Input: dimensioned drawing with shaded views. Units: mm. Origin: part minimum x, y, z. Give positions to 0.01 mm unless a question says otherwise; leave off trailing zeros. Write each loop counter-clockwise with the first axis right and the second up, starting at its lowest first coordinate (ties: lowest second). Pieces come first, ordered by that corner, then holes.
Q1. Section A-A (y = 19). Return the cut outline in (x, z).
Q2. Pin query (flat end, axial travel): pin 1 Ø4 at (y, z) = (28.5, 11.5) entering from -X; pin 2 Ø5 at (y, z) = (26.5, 7.5) entering from -X; pin 3 Ø5 at (x, z) = (24.5, 17) entering from -Y. Return the tip coordinate at first contact, or that it passes through.
Q3. Mould query, pull axis Y, two halves, no side actions, for the marked faces 1, 2 and 3. Classes: +Y half, -Y half, draft (parallel to the pull), parting line (faces both ways), or undercut.
Q4. Line query: line 1 (Y direction, x = 19, z = 6.75); line 2 (Y direction, x = 14.5, z = 9.25); line 3 (X direction, y = 23, z = 12.5). Output: solid intervals per line, ascending.
Q5. Section C-C (z = 11.5). Return the cut outline in (x, y), plus the area to 3 significant figures.
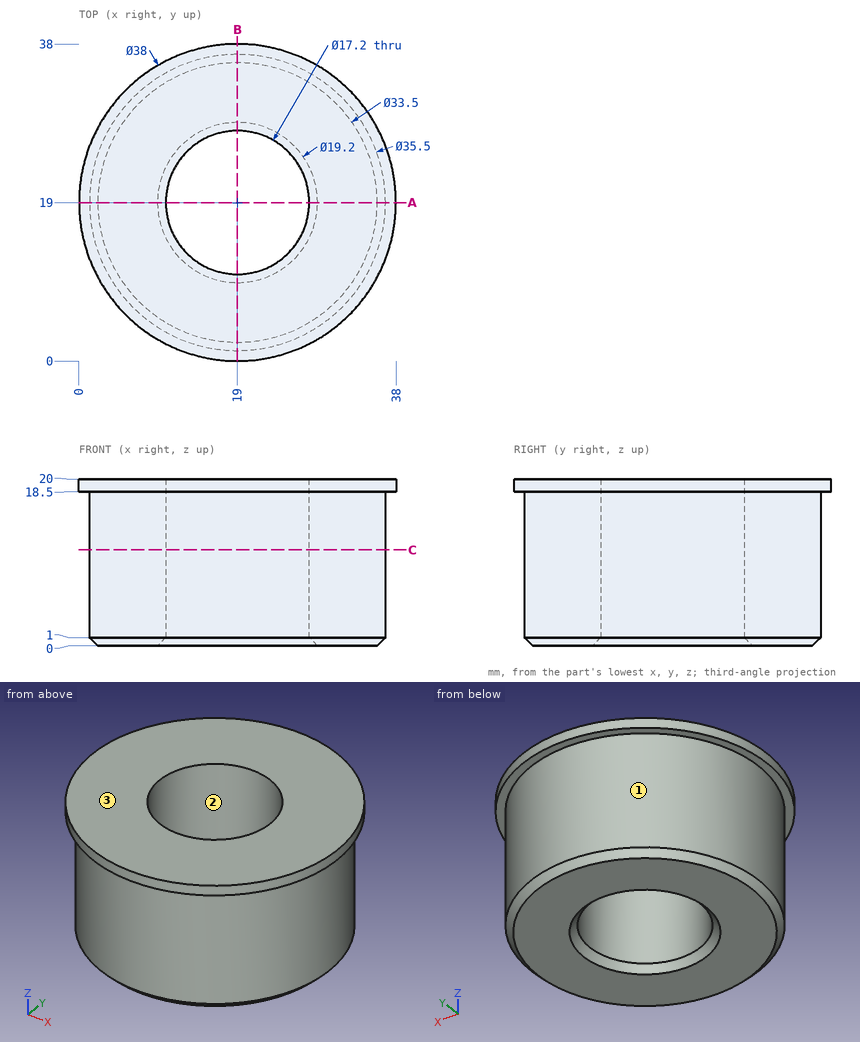
Computed:
1. outline: (0, 18.5) - (1.25, 18.5) - (1.25, 1) - (2.25, 0) - (9.4, 0) - (10.4, 1) - (10.4, 20) - (0, 20) - close; (27.6, 1) - (28.6, 0) - (35.75, 0) - (36.75, 1) - (36.75, 18.5) - (38, 18.5) - (38, 20) - (27.6, 20) - close
2. pin 1: stops at x = 2.91
2. pin 2: stops at x = 1.97
2. pin 3: stops at y = 0.33
3. face 1: parting line
3. face 2: undercut
3. face 3: draft
4. line 1: y = 1.25 to 10.4, 27.6 to 36.75
4. line 2: y = 1.83 to 11.67, 26.33 to 36.17
4. line 3: x = 1.71 to 11.39, 26.61 to 36.29
5. outline: circle Ø35.5 at (19, 19); hole circle Ø17.2 at (19, 19)
5. area: 757 mm2
